Geometry: see drawing. Coordinates: mm, zero at the bounding-box minimum. A direction names the side the tool comes from. Round coordinates to 2 decimals unless told otherwise and drop trailing zeros. Write each loop counter-clockwise with the first axis right and the second up, starting at its lowest first coordinate (ties: lowest second). Pieces come first, ordered by that corner, then holes. Notation, with made-up numbers: M -2,70 L 39,70 A36 ccw 39,105 Z; hole C 41.5,72.5 d11. An arc over 180 degrees is marked long. Use one line per item in the form item = value. Start each with the question number.
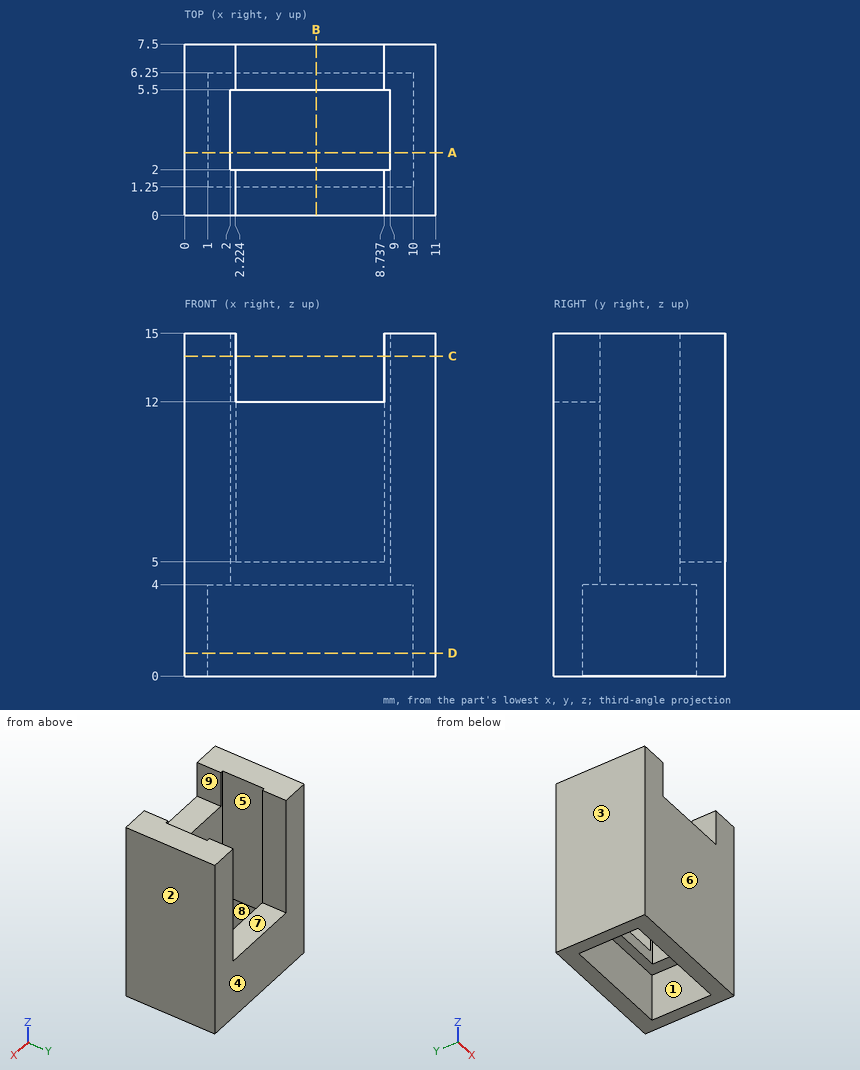
Item 1: Cut plane A-A (y = 2.75). Output: boundary loops of the cut face in (x, z), plus the area to 3 significant figures.
Item 2: Cut plane C-C (z = 14). Output: boundary loops of the cut face in (x, y).
Item 3: Reachability of the marked faces 5, 6, 7, 8 and 9 from +Z, -Z, +X, -X, +Y, -Y: full face, straight path, thin tool, end or side. Return the list, or none.
Item 4: First-contact query: pin 1 (3.5 mm diameter, centred on x = 4.5, z = 8, fed in from +Y); pin 2 (1 mm diameter, centred on x = 4.5, y = 1.5, fed in from +Z). Flat tips, straight axial feed; report the tip coordinate or a pass-through.
Item 5: Draft query along X for the marked faces 1, 2, 3 and 4. Return one class per face: +X half, -X half, draft (parallel to the pull), parting line (faces both ways), or undercut.
Item 6: Ray query, line 1 (X direction, y = 4.25, z = 14); line 2 (Y direction, x = 7.25, z = 1); line 3 (X direction, y = 5.5, z = 1.5). Return the intervals inside material, ascending. Write a range as from..to.
Item 7: Cut plane D-D (z = 1). Output: boundary loops of the cut face in (x, y), plus the area to 3 significant figures.
Item 8: Cut plane B-B (x = 5.75). Output: boundary loops of the cut face in (y, z).
Final values:
q1.outline = M 0,0 L 1,0 L 1,4 L 2,4 L 2,15 L 0,15 Z; M 9,4 L 10,4 L 10,0 L 11,0 L 11,15 L 9,15 Z
q1.area = 52.0 mm^2
q2.outline = M 0,0 L 2.22,0 L 2.22,2 L 2,2 L 2,5.5 L 2.22,5.5 L 2.22,7.5 L 0,7.5 Z; M 8.74,0 L 11,0 L 11,7.5 L 8.74,7.5 L 8.74,5.5 L 9,5.5 L 9,2 L 8.74,2 Z
q3.face_5 = +Z, -Z
q3.face_6 = +Z, -Z, +X, -X, -Y
q3.face_7 = +Z, +Y
q3.face_8 = -Z
q3.face_9 = +Z, +Y, -Y
q4.pin_1 = 2
q4.pin_2 = 12
q5.face_1 = undercut
q5.face_2 = +X half
q5.face_3 = -X half
q5.face_4 = draft
q6.line_1 = 0..2, 9..11
q6.line_2 = 0..1.25, 6.25..7.5
q6.line_3 = 0..1, 10..11
q7.outline = M 0,0 L 11,0 L 11,7.5 L 0,7.5 Z; hole M 1,1.25 L 10,1.25 L 10,6.25 L 1,6.25 Z
q7.area = 37.5 mm^2
q8.outline = M 0,0 L 1.25,0 L 1.25,4 L 2,4 L 2,12 L 0,12 Z; M 5.5,4 L 6.25,4 L 6.25,0 L 7.5,0 L 7.5,5 L 5.5,5 Z
